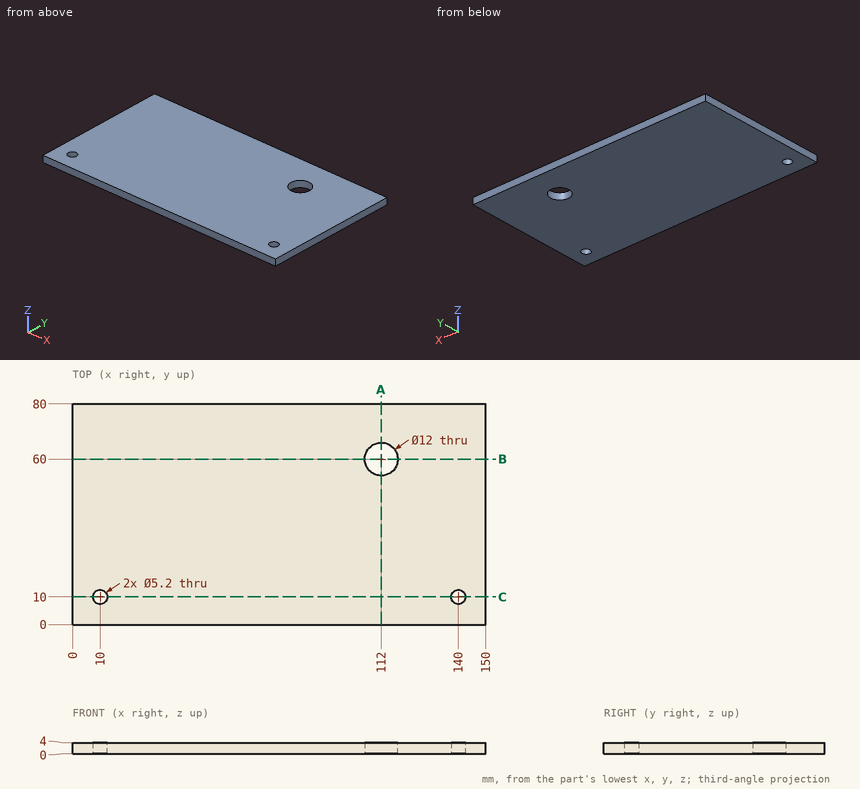
For this review, use the dimensioned drawing (mm, ordinates from the lowest corner) and the shaded views. Round coordinates to 2 decimals unless told otherwise and drop trailing zeros. Order: outer loops, then holes, each group sorted by start corner. A loop starts at its lowest first (then second) coordinate and runs counter-clockwise, first axis right, second up.
1) Consider section C-C (y = 10). State the section outline as (x, z) points.
The answers:
outline: (0, 0) - (7.4, 0) - (7.4, 4) - (0, 4) - close; (12.6, 0) - (137.4, 0) - (137.4, 4) - (12.6, 4) - close; (142.6, 0) - (150, 0) - (150, 4) - (142.6, 4) - close
2) Clearance check with a flat-ended pin moving along its axis: pin 1 Ø9.5 at (x, y) = (112, 60) entering from +Z. State where the tip first meets the part, or that it passes through.
The answers:
pin 1: passes through
3) Consider section B-B (y = 60). State the section outline as (x, z) points.
The answers:
outline: (0, 0) - (106, 0) - (106, 4) - (0, 4) - close; (118, 0) - (150, 0) - (150, 4) - (118, 4) - close
4) Consider section A-A (x = 112). State the section outline as (y, z) points, plus the area to 3 significant figures.
The answers:
outline: (0, 0) - (54, 0) - (54, 4) - (0, 4) - close; (66, 0) - (80, 0) - (80, 4) - (66, 4) - close
area: 272 mm2
5) For L1, parallel to X at y = 10, z = 1.55; L2, parallel to Y at x = 10, z = 0.4; L3, parallel to Y at x = 112, z = 1.5, list the stretches that pass through material, from the lowest coordinate up.
The answers:
L1: x = 0 to 7.4, 12.6 to 137.4, 142.6 to 150
L2: y = 0 to 7.4, 12.6 to 80
L3: y = 0 to 54, 66 to 80
